Autodesk Inventor part; units mm, degrees
ref_plane "YZ Plane" through (0, 0, 0) normal (1, 0, 0) x (0, 1, 0)
ref_plane "XZ Plane" through (0, 0, 0) normal (0, 1, 0) x (-1, 0, 0)
ref_plane "XY Plane" through (0, 0, 0) normal (0, 0, 1) x (1, 0, 0)
sketch "Sketch1" plane through (0, 0, 0) normal (0, 1, 0) x (-1, 0, 0)
  line L0 (0, 0) -> (50.8, 0)
  line L1 (50.8, 0) -> (50.8, -50.8)
  line L2 (50.8, -50.8) -> (0, -50.8)
  line L3 (0, -50.8) -> (0, 0)
  dimension "d0" = 50.8
  dimension "d1" = 50.8
extrude "Extrusion1" add sketch "Sketch1" along normal blind 25.4
sketch "Sketch2" plane through (-50.8, 0, 0) normal (0, 0, 1) x (1, 0, 0)
  line L0 (50.8, 0) -> (0, 0) construction
  line L1 (50.8, 0) -> (31.75, 0) construction
  line L2 (31.75, 0) -> (31.75, 12.7) construction
  line L3 (31.75, 12.7) -> (50.8, 12.7) construction
  line L4 (50.8, 12.7) -> (50.8, 0) construction
  circle A0 centre (31.75, 12.7) radius 6.35
  dimension "d4" = 19.05
  dimension "d5" = 12.7
  dimension "d6" = 12.7
extrude "Extrusion2" cut sketch "Sketch2" against normal blind 66.675
sketch "Sketch3" plane through (0, 25.4, 0) normal (0, 1, 0) x (1, 0, 0)
  line L0 (-50.8, 0) -> (-35.56, 0) construction
  line L1 (-35.56, 0) -> (-35.56, 25.4) construction
  line L2 (-35.56, 25.4) -> (-50.8, 25.4) construction
  line L3 (-50.8, 25.4) -> (-50.8, 0) construction
  circle A0 centre (-35.56, 25.4) radius 9.525
  point P0 (0, 0)
  dimension "d9" = 15.24
  dimension "d10" = 25.4
  dimension "d11" = 19.05
extrude "Extrusion3" cut sketch "Sketch3" against normal blind 31.75
properties part number "AxleToRodAdapter"
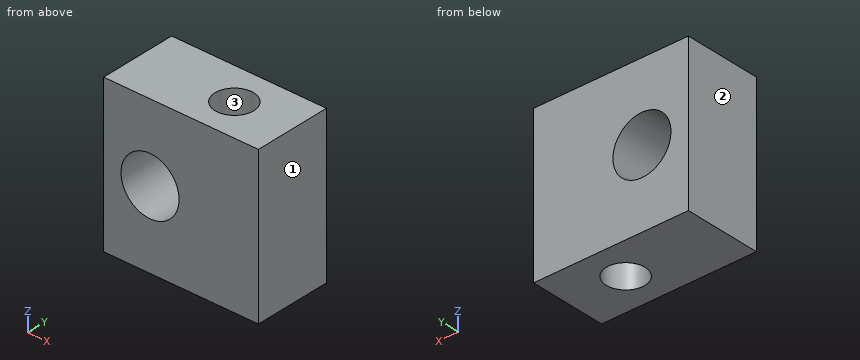
Build history of the part. All positions in model axes, mm. Face numbers are marked on the shaded views. Round coordinates to 2 decimals unless told otherwise and drop trailing zeros. Write each loop counter-clockwise with the first axis right and the second up, starting at its lowest first coordinate (ties: lowest second). Pieces come first, ordered by that corner, then holes. Notation, with made-up numbers: (72.5, 28) - (124.5, 28) arc R27 ccw to (124.5, 63) - close; hole circle Ø8 at (5, -18). An arc over 180 degrees is marked (long way). Answer as CSV lines item,"result".
Q1. Cut at B-B (y = 12.7). Write the cut outline in (x, z) (3 decimals).
Report:
outline,"(-50.8, -50.8) - (-25.4, -50.8) - (-25.4, 0) - (-50.8, 0) - close; (-12.7, -50.8) - (0, -50.8) - (0, 0) - (-12.7, 0) - close; hole circle Ø19.05 at (-35.56, -25.4)"
Q2. Drill centre lines: probe 1 along X at (y, z) = (14, -25); probe 2 along X at (y, z) = (10.25, -23); probe 3 along Y at (x, z) = (-19.05, -17). Where is each one in solid material? Low to high. Write a range as [from, to].
Report:
probe 1,"x = [-50.8, -45.08], [-26.04, -25.27], [-12.83, 0]"
probe 2,"x = [-50.8, -44.78], [-26.34, -24.91], [-13.19, 0]"
probe 3,"y = [0, 6.35], [19.05, 25.4]"
Q3. Pull direction X, two halves, no side cores. Call the marked faces 1, 2 and 3: +X half, -X half, draft (parallel to the pull), parting line (faces both ways), or undercut.
Report:
face 1,"+X half"
face 2,"-X half"
face 3,"undercut"
Q4. Cut at C-C (z = -34). Write the cut outline in (x, y), and give its area (3 significant figures).
Report:
outline,"(-50.8, 0) - (-39.65, 0) - (-39.65, 25.4) - (-50.8, 25.4) - close; (-31.47, 0) - (0, 0) - (0, 25.4) - (-31.47, 25.4) - close; hole circle Ø12.7 at (-19.05, 12.7)"
area,"956 mm^2"
Q5. Cut at A-A (x = -35.56). Write the cut outline in (y, z) (3 decimals), and give its area (3 significant figures).
Report:
outline,"(0, -50.8) - (25.4, -50.8) - (25.4, -34.925) - (0, -34.925) - close; (0, -15.875) - (25.4, -15.875) - (25.4, 0) - (0, 0) - close"
area,"806 mm^2"
Q6. Cut at D-D (y = 21.75). Write the cut outline in (x, z) (3 decimals), and give its area (3 significant figures).
Report:
outline,"(-50.8, -50.8) - (0, -50.8) - (0, 0) - (-50.8, 0) - close; hole circle Ø19.05 at (-35.56, -25.4)"
area,"2,300 mm^2"
